Here's the drawing with two shaded views (mm, measured from the low corner). I have some questions. Round coordinates to 2 decimals unless told otherwise and drop trailing zeros. Order: outer loops, then holes, each group sorted by start corner. A loop starts at its lowest first (then second) coordinate and runs counter-clockwise, first axis right, second up.
Q1. Will these pins go through, and if not, where does the flat tip stop? P1, Ø1.5, axis at y = 14, z = 73.5, coming from the +X side; P2, Ø3, axis at x = 8, z = 87, coming from the +Y side; P3, Ø12, axis at x = 10, y = 16.5, coming from the -Z side; P4, Ø1.5, axis at y = 11.5, z = 81.5, coming from the -X side.
Q2. If we section it at D-D (z = 106): Please give me the cut outline in (x, y), plus the area to 3 significant figures.
Q3. If we section it at A-A (y = 17.75): Please give me the cut outline in (x, z).
Q4. If I drill on line 1 (Z direction, x = 1, y = 18.25); line 2 (X direction, y = 14.75, z = 57), over which ranges is the centre line in solid material (lowest first)?
Q5. If we section it at C-C (y = 8.5): Please give me the cut outline in (x, z), plus the area to 3 significant figures.
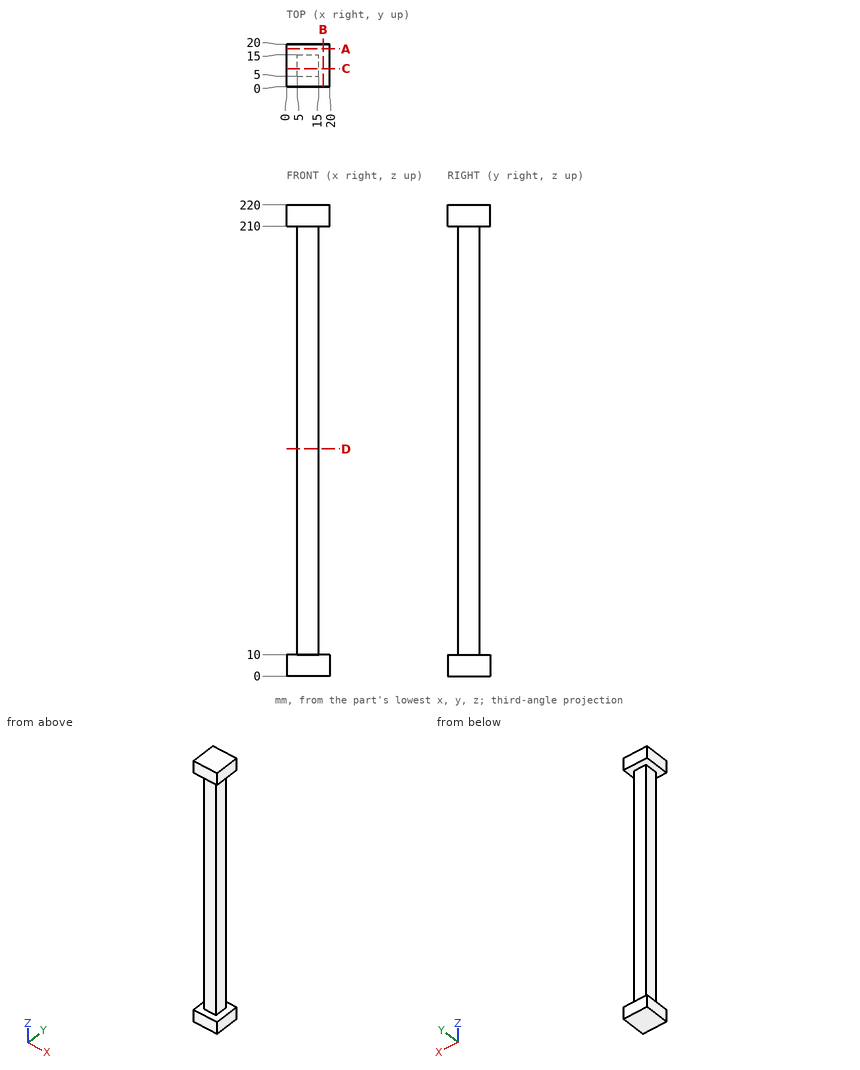
Solution:
1. P1: stops at x = 15
1. P2: stops at y = 15
1. P3: stops at z = 0
1. P4: stops at x = 5
2. outline: (5, 5) - (15, 5) - (15, 15) - (5, 15) - close
2. area: 100 mm2
3. outline: (0, 0) - (20, 0) - (20, 10) - (0, 10) - close; (0, 210) - (20, 210) - (20, 220) - (0, 220) - close
4. line 1: z = 0 to 10, 210 to 220
4. line 2: x = 5 to 15
5. outline: (0, 0) - (20, 0) - (20, 10) - (15, 10) - (15, 210) - (20, 210) - (20, 220) - (0, 220) - (0, 210) - (5, 210) - (5, 10) - (0, 10) - close
5. area: 2,400 mm2
